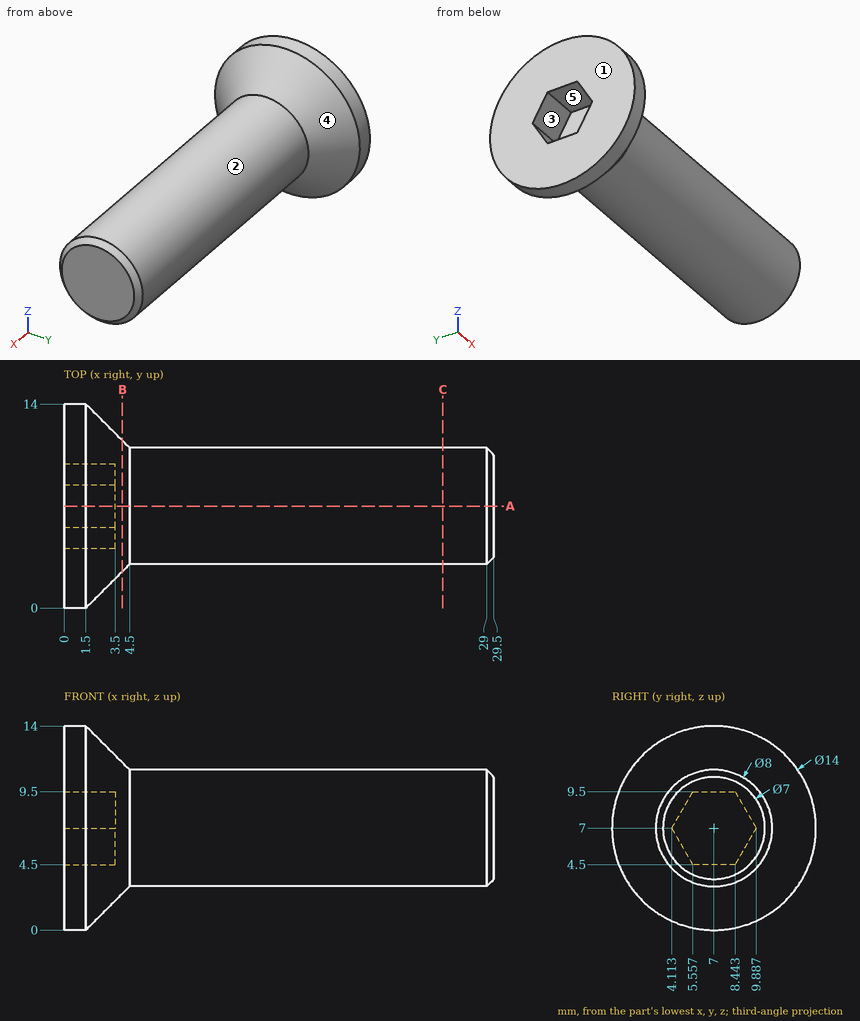
Verification items for this drawing (mm, ordinates from the low corner). A direction names the side the tool comes from. Coordinates: 2 decimals unless noted, no trailing zeros. Order: outer loops, then holes, each group sorted by start corner. A loop starts at its lowest first (then second) coordinate and runs counter-clockwise, first axis right, second up. Notation, with made-up numbers: (49, 31.25) -> (59, 31.25) arc R19 ccw to (59, 53.25) -> close; hole circle Ø9 at (30.5, 8.5). An arc over 180 degrees is marked (long way). Answer as CSV lines item,"result". Start each with the question number.
1) Gauge pin test, flat ends, axial feed: pin 1 Ø5 at (x, z) = (22, 11.5) entering from -Y (1 decimal); pin 2 Ø1 at (x, y) = (21.5, 6) entering from -Z; pin 3 Ø6 at (x, y) = (15, 12.5) entering from -Z. Record the tip position at first contact, or that the pin passes through.
2) Cross-section at A-A, the plane y = 7. Record the boundary of the cut face in (x, z), then the cut area to 3 significant figures.
3) Cross-section at B-B, the plane x = 4. Record the boundary of the cut face in (y, z), then the cut area to 3 significant figures.
4) Set-up check for the marked faces 4 and 5: record each of +Z, -Z, +X, -X, +Y, -Y from which the full face is reachable in a straight line by a thin tool's end or side.
5) Release check for a two-part mould opening along Z. For the marked faces 1, 2 and 3 record: released by +Z, released by -Z, zero draft, split by the parting line, or undercut.
6) Cross-section at C-C, the plane x = 26. Record the boundary of the cut face in (y, z).
7) Material ranges on L1, parallel to Y at x = 23.5, z = 7; L2, parallel to Z at x = 18, y = 10 (1 decimal); L3, parallel to Y at x = 3.75, z = 8 (1 decimal), recorded low to high. Write a range as [from, to].
Conclusion:
1,pin 1,"stops at y = 3.5"
1,pin 2,"stops at z = 3.03"
1,pin 3,"stops at z = 3.88"
2,outline,"(0, 0) -> (1.5, 0) -> (4.5, 3) -> (29, 3) -> (29.5, 3.5) -> (29.5, 10.5) -> (29, 11) -> (4.5, 11) -> (1.5, 14) -> (0, 14) -> (0, 9.5) -> (3.5, 9.5) -> (3.5, 4.5) -> (0, 4.5) -> close"
2,area,"236 mm²"
3,outline,"circle Ø9 at (7, 7)"
3,area,"63.6 mm²"
4,face 4,"+X"
4,face 5,"-X"
5,face 1,"zero draft"
5,face 2,"split by the parting line"
5,face 3,"undercut"
6,outline,"circle Ø8 at (7, 7)"
7,L1,"y = [3, 11]"
7,L2,"z = [4.4, 9.6]"
7,L3,"y = [2.4, 11.6]"
